Drawing for the job (mm, zero at the part's lowest x, y, z). A direction names the side the tool comes from. Give positions to 0.01 mm unless a question says otherwise; leave off trailing zeros. Write each loop counter-clockwise with the first axis right and the second up, starting at its lowest first coordinate (ties: lowest second). Pieces come first, ordered by that corner, then holes. Notation, with made-up numbers: M 75,-3 L 111,-3 A20 ccw 111,24 Z; hole C 30,48.25 d6. An arc over 180 degrees is marked long. Use a Markdown table: item, result. Add a question column.
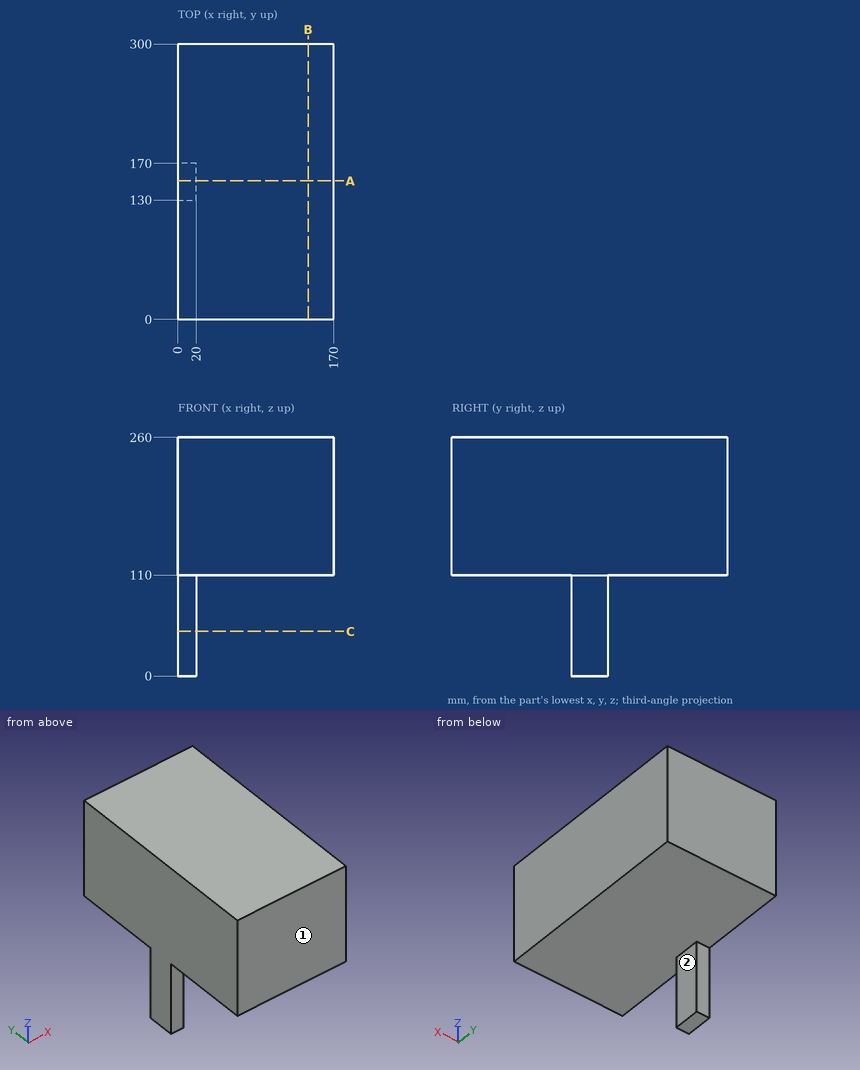
1. Flat gauge pins, fed straight in: pin 1 (10 mm diameter, centred on x = 116.5, y = 260.5, fed in from -Z); pin 2 (10 mm diameter, centred on x = 9, z = 34.5, fed in from +Y); pin 3 (12 mm diameter, centred on y = 158, z = 42, fed in from +X). Where does each tip first touch, or does it go through?
2. Cut at A-A (y = 151). Write the cut outline in (x, z), then the cut area to 3 significant figures.
3. Cut at B-B (x = 142). Write the cut outline in (y, z), then the cut area to 3 significant figures.
4. Cut at C-C (z = 48.5). Write the cut outline in (x, y), then the cut area to 3 significant figures.
5. Drill centre line: probe 1 along Z at (x, y) = (14, 181). Where is it in solid material? Low to high. Write a range as [from, to].
6. Tool access for the marked faces 1 and 2: list every direction of +Z, -Z, +X, -X, +Y, -Y with a clear straight run to the whole face (end or side of a thin tool).
A:
| question | item | result |
|---|---|---|
| 1 | pin 1 | stops at z = 110 |
| 1 | pin 2 | stops at y = 170 |
| 1 | pin 3 | stops at x = 20 |
| 2 | outline | M 0,0 L 20,0 L 20,110 L 170,110 L 170,260 L 0,260 Z |
| 2 | area | 27,700 mm² |
| 3 | outline | M 0,110 L 300,110 L 300,260 L 0,260 Z |
| 3 | area | 45,000 mm² |
| 4 | outline | M 0,130 L 20,130 L 20,170 L 0,170 Z |
| 4 | area | 800 mm² |
| 5 | probe 1 | z = [110, 260] |
| 6 | face 1 | +Z, -Z, +X, -X, -Y |
| 6 | face 2 | -Z, +X, +Y, -Y |
